```python
from build123d import *

# Parameters (mm, degrees)
BOSS_EXTRUDE1_DEPTH = 3.175
CUT_EXTRUDE4_DEPTH  = 235.179100055
SKETCH5_R           = 2.54
CUT_EXTRUDE3_DEPTH  = 235.179100055
SKETCH4_R           = 2.159
CUT_EXTRUDE2_DEPTH  = 235.179100055
FILLET1_R           = 25.4
SKETCH6_W           = 3.81
SKETCH6_H           = 6.985
CUT_EXTRUDE5_DEPTH  = 235.179100055


with BuildPart() as part:
    # Sketch1 → Boss-Extrude1 (new body)
    with BuildSketch(Plane(origin=(0, 0, 0), x_dir=(1, 0, 0), z_dir=(0, 1, 0))):
        Polygon((-139.7, 73.520142619), (-121.739487758, 91.480654861), (121.739487758, 91.480654861), (139.7, 73.520142619), (139.7, -169.958832897), (121.739487758, -187.919345139), (-121.739487758, -187.919345139), (-139.7, -169.958832897), align=None)
    extrude(amount=BOSS_EXTRUDE1_DEPTH)

    # Sketch2 → Cut-Extrude4 (cut, through all)
    with BuildSketch(Plane(origin=(0, 3.175, 0), x_dir=(1, 0, 0), z_dir=(0, 1, 0))):
        Polygon((-103.778975516, 37.599118134), (-114.3, 27.07809365), (-114.3, -123.516783928), (-103.778975516, -134.037808413), (-85.818463274, -151.998320655), (-75.297438789, -162.519345139), (75.297438789, -162.519345139), (85.818463274, -151.998320655), (103.778975516, -134.037808413), (114.3, -123.516783928), (114.3, 27.07809365), (103.778975516, 37.599118134), (85.818463274, 55.559630377), (75.297438789, 66.080654861), (-75.297438789, 66.080654861), (-85.818463274, 55.559630377), align=None)
    extrude(amount=-CUT_EXTRUDE4_DEPTH, mode=Mode.SUBTRACT)

    # Sketch5 → Cut-Extrude3 (cut, through all)
    with BuildSketch(Plane(origin=(0, 3.175, 0), x_dir=(1, 0, 0), z_dir=(0, 1, 0))):
        with Locations(Location((-121.739487758, 73.520142619, 0), (0, 0, 270))):
            Circle(SKETCH5_R)
        with Locations(Location((-103.778975516, 55.559630377, 0), (0, 0, 270))):
            Circle(SKETCH5_R)
        with Locations(Location((103.778975516, 55.559630377, 0), (0, 0, 90))):
            Circle(SKETCH5_R)
        with Locations(Location((121.739487758, 73.520142619, 0), (0, 0, 90))):
            Circle(SKETCH5_R)
        with Locations(Location((121.739487758, -169.958832897, 0), (0, 0, 270))):
            Circle(SKETCH5_R)
        with Locations(Location((103.778975516, -151.998320655, 0), (0, 0, 270))):
            Circle(SKETCH5_R)
        with Locations(Location((-103.778975516, -151.998320655, 0), (0, 0, 90))):
            Circle(SKETCH5_R)
        with Locations(Location((-121.739487758, -169.958832897, 0), (0, 0, 90))):
            Circle(SKETCH5_R)
    extrude(amount=-CUT_EXTRUDE3_DEPTH, mode=Mode.SUBTRACT)

    # Sketch4 → Cut-Extrude2 (cut, through all)
    with BuildSketch(Plane(origin=(0, 3.175, 0), x_dir=(1, 0, 0), z_dir=(0, 1, 0))):
        with Locations(Location((0, 81.320654861, 0), (0, 0, 270))):
            Circle(SKETCH4_R)
        with Locations(Location((-44.45, 81.320654861, 0), (0, 0, 270))):
            Circle(SKETCH4_R)
        with Locations(Location((44.45, 81.320654861, 0), (0, 0, 270))):
            Circle(SKETCH4_R)
        with Locations(Location((-22.225, 81.320654861, 0), (0, 0, 270))):
            Circle(SKETCH4_R)
        with Locations(Location((22.225, 81.320654861, 0), (0, 0, 270))):
            Circle(SKETCH4_R)
        with Locations(Location((-129.54, -48.219345139, 0), (0, 0, 270))):
            Circle(SKETCH4_R)
        with Locations(Location((-129.54, -25.994345139, 0), (0, 0, 270))):
            Circle(SKETCH4_R)
        with Locations(Location((-129.54, -3.769345139, 0), (0, 0, 270))):
            Circle(SKETCH4_R)
        with Locations(Location((129.54, -48.219345139, 0), (0, 0, 270))):
            Circle(SKETCH4_R)
        with Locations(Location((129.54, -25.994345139, 0), (0, 0, 270))):
            Circle(SKETCH4_R)
        with Locations(Location((129.54, -3.769345139, 0), (0, 0, 270))):
            Circle(SKETCH4_R)
        with Locations(Location((129.54, -92.669345139, 0), (0, 0, 90))):
            Circle(SKETCH4_R)
        with Locations(Location((129.54, -70.444345139, 0), (0, 0, 90))):
            Circle(SKETCH4_R)
        with Locations(Location((-129.54, -92.669345139, 0), (0, 0, 90))):
            Circle(SKETCH4_R)
        with Locations(Location((-129.54, -70.444345139, 0), (0, 0, 90))):
            Circle(SKETCH4_R)
        with Locations(Location((22.225, -177.759345139, 0), (0, 0, 90))):
            Circle(SKETCH4_R)
        with Locations(Location((-22.225, -177.759345139, 0), (0, 0, 90))):
            Circle(SKETCH4_R)
        with Locations(Location((44.45, -177.759345139, 0), (0, 0, 90))):
            Circle(SKETCH4_R)
        with Locations(Location((-44.45, -177.759345139, 0), (0, 0, 90))):
            Circle(SKETCH4_R)
        with Locations(Location((0, -177.759345139, 0), (0, 0, 90))):
            Circle(SKETCH4_R)
        with Locations(Location((-66.675, 81.320654861, 0), (0, 0, 270))):
            Circle(SKETCH4_R)
        with Locations(Location((66.675, 81.320654861, 0), (0, 0, 270))):
            Circle(SKETCH4_R)
        with Locations(Location((-129.54, 18.455654861, 0), (0, 0, 270))):
            Circle(SKETCH4_R)
        with Locations(Location((129.54, 18.455654861, 0), (0, 0, 270))):
            Circle(SKETCH4_R)
        with Locations(Location((129.54, -114.894345139, 0), (0, 0, 90))):
            Circle(SKETCH4_R)
        with Locations(Location((66.675, -177.759345139, 0), (0, 0, 90))):
            Circle(SKETCH4_R)
        with Locations(Location((-66.675, -177.759345139, 0), (0, 0, 90))):
            Circle(SKETCH4_R)
        with Locations(Location((-129.54, -114.894345139, 0), (0, 0, 90))):
            Circle(SKETCH4_R)
        with Locations(Location((-129.54, -137.119345139, 0), (0, 0, 270))):
            Circle(SKETCH4_R)
        with Locations(Location((-129.54, 40.680654861, 0), (0, 0, 90))):
            Circle(SKETCH4_R)
        with Locations(Location((129.54, 40.680654861, 0), (0, 0, 270))):
            Circle(SKETCH4_R)
        with Locations(Location((129.54, -137.119345139, 0), (0, 0, 90))):
            Circle(SKETCH4_R)
    extrude(amount=-CUT_EXTRUDE2_DEPTH, mode=Mode.SUBTRACT)

    # Fillet1
    fillet1_edges = [part.edges().sort_by_distance(p)[0] for p in [
        (-75.297438789, 1.5875, -66.080654861),
        (75.297438789, 1.5875, -66.080654861),
        (114.3, 1.5875, -27.07809365),
        (114.3, 1.5875, 123.516783928),
        (75.297438789, 1.5875, 162.519345139),
        (-75.297438789, 1.5875, 162.519345139),
        (-114.3, 1.5875, 123.516783928),
        (-114.3, 1.5875, -27.07809365),
    ]]
    fillet(fillet1_edges, radius=FILLET1_R)

    # Sketch6 → Cut-Extrude5 (cut, through all)
    with BuildSketch(Plane(origin=(0, 3.175, 0), x_dir=(1, 0, 0), z_dir=(0, 1, 0))):
        with Locations((-137.795, 7.343154861)):
            Rectangle(SKETCH6_W, SKETCH6_H)
        with Locations((-137.795, -103.781845139)):
            Rectangle(SKETCH6_W, SKETCH6_H)
        with Locations((137.795, -103.781845139)):
            Rectangle(SKETCH6_W, SKETCH6_H)
        with Locations((137.795, 7.343154861)):
            Rectangle(SKETCH6_W, SKETCH6_H)
    extrude(amount=-CUT_EXTRUDE5_DEPTH, mode=Mode.SUBTRACT)


solid = part.part
```
The model under review builds one solid part; all positions refer to its coordinate system, in mm. A direction names the side the tool comes from. Round coordinates to 2 decimals unless told otherwise and drop trailing zeros. Loops run counter-clockwise (first coordinate to the right, second up) from the corner with the lowest first, then second, coordinate; pieces in that order, holes last. Notation, with made-up numbers: M 5,38 L 30,38 A8 ccw 30,51 Z; hole C 14.25,-24 d10. An arc over 180 degrees is marked long. Answer as a JSON object with one key per item and string values.
(1) Draft analysis for pull direction X (two halves, no side actions). For faces 1 (the flat face through (-130.85, 1.57, -82.37)), 2 (the cylindrical face through (-74.63, 1.57, -64.09)), 3 (the flat face through (130.85, 1.57, 178.81)), 4 (the flat face through (126, 3.175, 46)), state which applies: released by +X, released by -X, zero draft, split by the parting line, or undercut.
Resolved:
{"face 1": "released by -X", "face 2": "undercut", "face 3": "released by +X", "face 4": "zero draft"}
(2) Take a section at A-A on x = 28.5. Give the boundary of the cut face in (y, z) (3 decimals), and give its area (3 significant figures).
Resolved:
{"outline": "M 0,-91.481 L 3.175,-91.481 L 3.175,-66.081 L 0,-66.081 Z; M 0,162.519 L 3.175,162.519 L 3.175,187.919 L 0,187.919 Z", "area": "161 mm²"}
(3) Take a section at C-C on y = 1.2. Count the separate pieces of the cut face and the enclosed holes in it, and give its area (3 significant figures).
Resolved:
{"separate pieces": "1", "enclosed holes": "41", "area": "27,600 mm²"}
(4) Take a section at B-B on z = 13.5. Give the boundary of the cut face in (x, y) (3 decimals).
Resolved:
{"outline": "M -139.7,0 L -114.3,0 L -114.3,3.175 L -139.7,3.175 Z; M 114.3,0 L 139.7,0 L 139.7,3.175 L 114.3,3.175 Z"}
(5) To check wall thickness, follow line 1 along X through (y, z) = (1.55, 169.5); line 2 along Z through (x, y) = (-25.5, 1.55); line 3 along X through (y, z) = (3, 49). State the ranges of each line that lie inside material, in increasing order.
Resolved:
{"line 1": "-139.7 to -124.24, -119.24 to 119.24, 124.24 to 139.7", "line 2": "-91.48 to -66.08, 162.52 to 187.92", "line 3": "-139.7 to -131.55, -127.53 to -114.3, 114.3 to 127.53, 131.55 to 139.7"}
(6) Tool access review of faces 5 (the flat face through (-130.594, 1.565, 179.065)), 6 (the cylindrical face through (-74.63, 1.57, 160.53)): name each direction out of +Z, -Z, +X, -X, +Y, -Y from which nothing blocks a thin tool from reaching the whole face with its end or side.
Resolved:
{"face 5": "+Z, -X, +Y, -Y", "face 6": "+Y, -Y"}
(7) Clearance check with flat-ended pins moving along their axes: P1, Ø3.5, axis at x = -129.54, z = 114.89, coming from the -Y side; P2, Ø1, axis at y = 1, z = -10, coming from the +X side; P3, Ø1, axis at x = -137.5, y = 1.5, coming from the -Z side. State where each tip first meets the part, or that it passes through.
Resolved:
{"P1": "through", "P2": "x = 135.89", "P3": "z = -76.22"}
